Print and shaded views of the part. All mm, measured from the part's lowest x, y and z. A direction names the side the tool comes from. Round coordinates to 2 decimals unless told otherwise and drop trailing zeros. Order: outer loops, then holes, each group sorted by start corner. A loop starts at its lowest first (then second) coordinate and runs counter-clockwise, first axis right, second up. Notation, with made-up numbers: M -9.5,31 L 0.5,31 A19 ccw 0.5,62 Z; hole C 12.25,44.5 d11. An arc over 180 degrees is marked long. Write each question's results on one line, items separated by ' | '. Start each with the question number.
1. Band-saw the part on A-A, the plane x = 47. List the corners of the cut face in (y, z), then the cut area to 3 significant figures.
2. Which spindle directions (+Z, -Z, +X, -X, +Y, -Y) get a long thin tool onto all of the face, cutting with end or side? Do the marked faces 4 and 5. Say none if no direction does.
3. Drop a flat-ended pin along its axis: pin 1 Ø5 at (x, z) = (11, 5.5) entering from +Y. Give the stop position or say it passes through.
4. Band-saw the part on B-B, the plane y = 39.5. List the corners of the cut face in (x, z).
5. Band-saw the part on D-D, the plane y = 46. List the corners of the cut face in (x, z), then the cut area to 3 significant figures.
6. Two-plate mould, pull along X, no slides. Class the marked faces 1, 2 and 3: +X half, -X half, draft (parallel to the pull), parting line (faces both ways), or undercut.
7. Probe L1, parallel to Z at x = 31, y = 2; L2, parallel to Y at x = 6.45, z = 15.95; L3, parallel to Y at x = 33.5, z = 16.25. List the from-to ranges inside material, lowest first. Write a range as [from, to].
8. Band-saw the part on C-C, the plane x = 55.55. List the corners of the cut face in (y, z), then the cut area to 3 significant figures.
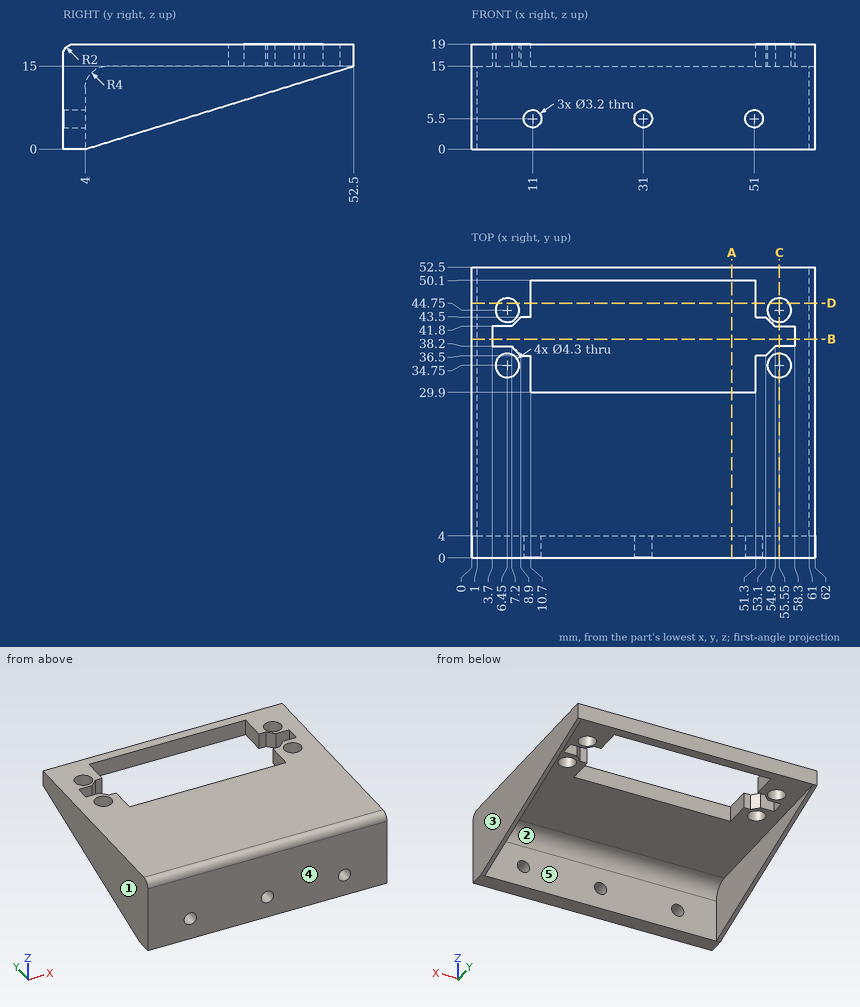
Solution:
1) outline: M 0,0 L 4,0 L 4,11 A4 cw 8,15 L 29.9,15 L 29.9,19 L 2,19 A2 ccw 0,17 Z; M 50.1,15 L 52.5,15 L 52.5,19 L 50.1,19 Z | area: 192 mm^2
2) face 4: +Z, -Z, +X, -X, -Y | face 5: -Z, +Y
3) pin 1: y = 4
4) outline: M 0,10.98 L 1,10.98 L 1,15 L 3.7,15 L 3.7,19 L 0,19 Z; M 58.3,15 L 61,15 L 61,10.98 L 62,10.98 L 62,19 L 58.3,19 Z
5) outline: M 0,12.99 L 1,12.99 L 1,15 L 4.7,15 L 4.7,19 L 0,19 Z; M 8.2,15 L 10.7,15 L 10.7,19 L 8.2,19 Z; M 51.3,15 L 53.8,15 L 53.8,19 L 51.3,19 Z; M 57.3,15 L 61,15 L 61,12.99 L 62,12.99 L 62,19 L 57.3,19 Z | area: 61.6 mm^2
6) face 1: -X half | face 2: undercut | face 3: +X half
7) L1: [0, 3.9], [7.1, 19] | L2: [0, 32.6], [36.9, 38.2], [41.8, 42.6], [46.9, 52.5] | L3: [0, 29.9], [50.1, 52.5]
8) outline: M 0,0 L 4,0 L 4,11 A4 cw 8,15 L 32.6,15 L 32.6,19 L 2,19 A2 ccw 0,17 Z; M 36.9,15 L 38.2,15 L 38.2,19 L 36.9,19 Z; M 41.8,15 L 42.6,15 L 42.6,19 L 41.8,19 Z; M 46.9,15 L 52.5,15 L 52.5,19 L 46.9,19 Z | area: 224 mm^2
